The listing builds one solid part. Answer for the finished solid, in the listing's coordinates (mm). Face numbers are marked on the shaded views. A direction names the side the tool comes from. Give positions to 0.01 mm unless a question says otherwise; leave off trailing zeros. Order: outer loops, then holes, each group sorted by start corner. A loop starts at its lowest first (then second) coordinate and runs counter-clockwise, first axis right, second up. Notation, with made-up numbers: (13.25, 0) - (39.25, 0) arc R12 cw to (39.25, 11) - close; hole circle Ø1 at (57.25, 33). An arc over 180 degrees is marked (long way). Answer as CSV lines item,"result". Start each with the question number.
1. Determine the mould class of the marked faces 3, 4, 5 and 6 for opening direction X: +X half, -X half, draft (parallel to the pull), parting line (faces both ways), or undercut.
2. Section D-D on z = 6 is taken. Count the separate pieces of the cut face and the enclosed holes in it, and give its area (3 significant figures).
3. Which of the six approach directions +Z, -Z, +X, -X, +Y, -Y give full straight-line access (tool end or side, diameter ignored) to the marked faces 1 and 2?
4. Section C-C on x = 11.5 is taken. Give the vertices of the cut face in (y, z) (3 decimals), and give its area (3 significant figures).
5. Section B-B on y = -18.5 is taken. Give the vertices of the cut face in (x, z) (3 decimals), and give its area (3 significant figures).
6. Flat-ended cylindrical pins translate along their axes: pin 1 (2.5 mm diameter, centred on y = -49, z = 6.5, fed in from +X); pin 2 (1 mm diameter, centred on x = 3.5, z = 11.5, fed in from -Y) (3 decimals); pin 3 (4 mm diameter, centred on y = -7.5, z = 21, fed in from +X) (3 decimals). Find the tip coordinate at first contact, or state that the pin passes through.
7. Section A-A on x = -23 is taken. Give the vertices of the cut face in (y, z) (3 decimals), and give its area (3 significant figures).
8. Consider line 1 along X through (y, z) = (-28, 5) (3 decimals); line 2 along Y through (x, z) = (29.5, 3) (3 decimals); line 3 along X through (y, z) = (3, 8.5) (3 decimals). Determine where each line is inside the solid, lowest interval first. Write a range as [from, to].
from build123d import *

# Parameters (mm, degrees)
F0_W     = 28
F0_H     = 8
F1_DEPTH = 10
F3_DEPTH = 25
F5_DEPTH = 10.001


with BuildPart() as f1:
    # F0 (on Top) → F1 (new body)
    with BuildSketch(Plane.XY):
        with Locations((0, -47.815)):
            Rectangle(F0_W, F0_H)
        Polygon((43.815, 15), (43.815, 43.815), (-43.815, 43.815), (-43.815, -43.815), (-14, -43.815), (-14, -35.815), (14, -35.815), (14, -43.815), (43.815, -43.815), (43.815, -15), (34.815, -15), (34.815, 15), align=None)
        with Locations((0, -39.815)):
            Rectangle(F0_W, F0_H)
    extrude(amount=F1_DEPTH)

    # F2 (on face) → F3 (join)
    with BuildSketch(Plane.XY.offset(10)):
        Polygon((43.815, 36.195), (43.815, 43.815), (-43.815, 43.815), (-43.815, -43.815), (-36.195, -43.815), (-36.195, 36.195), align=None)
    extrude(amount=F3_DEPTH)

    # F4 (on face) → F5 (cut, through all)
    with BuildSketch(Plane.XY.offset(10)):
        Polygon((-6.194999, 21.195), (-6.194999, 31.195), (-31.195, 31.195), (-31.195, -1.31), (-21.195, -1.31), (-21.195, 21.195), align=None)
        Polygon((38.815, 20), (38.815, 31.195), (4.814999, 31.195), (4.814999, 21.195), (19.815, 21.195), (19.815, -1.31), (29.815, -1.31), (29.815, 20), align=None)
        Polygon((14.814999, 16.194999), (4.814999, 16.194999), (4.814999, 6.194999), (4.814999, -1.31), (14.814999, -1.31), align=None)
        Polygon((-6.194999, 6.194999), (-6.194999, 16.194999), (-16.194999, 16.194999), (-16.194999, -1.31), (-6.194999, -1.31), align=None)
        Polygon((-6.194999, -6.31), (-16.194999, -6.31), (-16.194999, -23.814999), (-6.194999, -23.814999), (-6.194999, -13.814999), align=None)
        Polygon((-21.195, -6.31), (-31.195, -6.31), (-31.195, -38.815), (-9, -38.815), (-9, -46.815), (-6.194999, -46.815), (-6.194999, -28.815), (-21.195, -28.815), align=None)
        Polygon((29.815, -20), (29.815, -6.31), (19.815, -6.31), (19.815, -28.815), (4.814999, -28.815), (4.814999, -46.815), (9, -46.815), (9, -38.815), (38.815, -38.815), (38.815, -20), align=None)
        Polygon((14.814999, -23.814999), (14.814999, -6.31), (4.814999, -6.31), (4.814999, -13.814999), (4.814999, -23.814999), align=None)
    extrude(amount=-F5_DEPTH, mode=Mode.SUBTRACT)


solid = f1.part
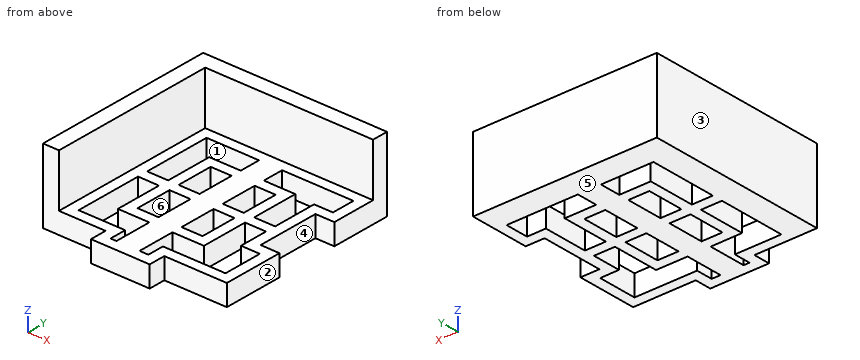
Checks:
1,face 3,"-X half"
1,face 4,"+X half"
1,face 5,"draft"
1,face 6,"undercut"
2,separate pieces,"1"
2,enclosed holes,"8"
2,area,"4,710 mm²"
3,face 1,"+Z, -Z"
3,face 2,"+Z, -Z, +X, +Y, -Y"
4,outline,"(-51.815, 0) - (-38.815, 0) - (-38.815, 10) - (-51.815, 10) - close; (-28.815, 0) - (-23.815, 0) - (-23.815, 10) - (-28.815, 10) - close; (-6.31, 0) - (-1.31, 0) - (-1.31, 10) - (-6.31, 10) - close; (16.195, 0) - (21.195, 0) - (21.195, 10) - (16.195, 10) - close; (31.195, 0) - (43.815, 0) - (43.815, 35) - (36.195, 35) - (36.195, 10) - (31.195, 10) - close"
4,area,"597 mm²"
5,outline,"(-43.815, 0) - (-31.195, 0) - (-31.195, 10) - (-36.195, 10) - (-36.195, 35) - (-43.815, 35) - close; (-21.195, 0) - (-16.195, 0) - (-16.195, 10) - (-21.195, 10) - close; (-6.195, 0) - (4.815, 0) - (4.815, 10) - (-6.195, 10) - close; (14.815, 0) - (19.815, 0) - (19.815, 10) - (14.815, 10) - close; (29.815, 0) - (43.815, 0) - (43.815, 10) - (29.815, 10) - close"
5,area,"667 mm²"
6,pin 1,"stops at x = 14"
6,pin 2,"stops at y = 36.195"
6,pin 3,"stops at x = -36.195"
7,outline,"(-43.815, 0) - (-38.815, 0) - (-38.815, 10) - (-43.815, 10) - close; (-6.31, 0) - (-1.31, 0) - (-1.31, 10) - (-6.31, 10) - close; (31.195, 0) - (43.815, 0) - (43.815, 35) - (36.195, 35) - (36.195, 10) - (31.195, 10) - close"
7,area,"417 mm²"
8,line 1,"x = [-43.815, -31.195], [-21.195, 19.815], [38.815, 43.815]"
8,line 2,"y = [-43.815, -38.815], [-6.31, -1.31], [31.195, 43.815]"
8,line 3,"x = [-43.815, -31.195], [-21.195, -16.195], [-6.195, 4.815], [14.815, 19.815], [29.815, 34.815]"
